```python
from build123d import *

# Parameters (mm, degrees)
SKETCH1_R               = 25
BOSS_EXTRUDE2_DEPTH     = 3.25
SKETCH2_R               = 4.5
BOSS_EXTRUDE3_DEPTH     = 10
SKETCH3_R               = 4.5
BOSS_EXTRUDE4_DEPTH     = 5
SKETCH4_R               = 3.1
CUT_EXTRUDE1_DEPTH      = 2.5
SKETCH6_R               = 1.875
CUT_EXTRUDE2_DEPTH      = 1
CUT_EXTRUDE2_DEPTH_BACK = 19.25


with BuildPart() as part:
    # Sketch1 → Boss-Extrude2 (new body, symmetric)
    with BuildSketch(Plane.XY):
        Circle(SKETCH1_R)
    extrude(amount=BOSS_EXTRUDE2_DEPTH, both=True)

    # Sketch2 → Boss-Extrude3 (add)
    with BuildSketch(Plane.XY):
        Circle(SKETCH2_R)
    extrude(amount=BOSS_EXTRUDE3_DEPTH)

    # Sketch3 → Boss-Extrude4 (add)
    with BuildSketch(Plane(origin=(0, 0, -3.25), x_dir=(-1, 0, 0), z_dir=(0, 0, -1))):
        Circle(SKETCH3_R)
    extrude(amount=BOSS_EXTRUDE4_DEPTH)

    # Sketch4 → Cut-Extrude1 (cut)
    with BuildSketch(Plane(origin=(0, 0, -8.25), x_dir=(-1, 0, 0), z_dir=(0, 0, -1))):
        Circle(SKETCH4_R)
    extrude(amount=-CUT_EXTRUDE1_DEPTH, mode=Mode.SUBTRACT)

    # Sketch6 → Cut-Extrude2 (cut, two sides)
    with BuildSketch(Plane.XY.offset(10)) as cut_extrude2_sk:
        Circle(SKETCH6_R)
    extrude(amount=CUT_EXTRUDE2_DEPTH, mode=Mode.SUBTRACT)
    extrude(cut_extrude2_sk.sketch, amount=-CUT_EXTRUDE2_DEPTH_BACK, mode=Mode.SUBTRACT)


solid = part.part
```
Design review of the part built by this model. Coordinates are the model's own, in mm. A direction names the side the tool comes from. Coordinates: 2 decimals unless noted, no trailing zeros. Write each loop counter-clockwise with the first axis right and the second up, starting at its lowest first coordinate (ties: lowest second). Pieces come first, ordered by that corner, then holes.
1) Add section A-A (x = 0). Write out the cut boundary in (y, z) (3 decimals), plus the area to 3 significant figures.
2) Machinability: for faces 1 (the flat face through (-1, -2, -5.75)), 2 (the cylindrical face through (23.846, 7.509, 0.046)), which of the approach directions +Z, -Z, +X, -X, +Y, -Y give a long, thin tool a straight path to every point of the face, cutting with its end or side? Answer none if there is none.
3) Insertion check: pin 1 (1 mm diameter, centred on y = -17.5, z = -3.5, fed in from -X); pin 2 (1.5 mm diameter, centred on x = -20, z = -5, fed in from +Y); pin 3 (5 mm diameter, centred on x = 0, y = 0, fed in from -Z); pin 4 (1.5 mm diameter, centred on y = -6, z = -2, fed in from +X). Each pin has a flat end and moves straight along its axis. Give the tip position at first contact, or say it passes through.
4) To check wall thickness, follow L1, parallel to Y at x = 0, z = -7.3; L2, parallel to Y at x = 0, z = 2.5 (3 decimals); L3, parallel to Z at x = 13, y = -4. State the ranges of each line that lie inside material, in increasing order.
5) Mouldability with a two-part tool opening along Y and no side actions: class faces 3 (the flat face through (0, -5, -3.25)), 4 (the cylindrical face through (-1.873, 0.082, 2.235)), 5 (the cylindrical face through (-0.59, 4.46, 6.58)) as +Y half, -Y half, draft (parallel to the pull), parting line (faces both ways), or undercut.
6) Add section C-C (z = -2.5). Write out the cut boundary in (x, y) (3 decimals), plus the area to 3 significant figures.
7) Add section D-D (x = -20). Write out the cut boundary in (y, z), plus the area to 3 significant figures.
Check result:
1. outline: (-25, -3.25) - (-4.5, -3.25) - (-4.5, -8.25) - (-3.1, -8.25) - (-3.1, -5.75) - (-1.875, -5.75) - (-1.875, 10) - (-4.5, 10) - (-4.5, 3.25) - (-25, 3.25) - close; (1.875, -5.75) - (3.1, -5.75) - (3.1, -8.25) - (4.5, -8.25) - (4.5, -3.25) - (25, -3.25) - (25, 3.25) - (4.5, 3.25) - (4.5, 10) - (1.875, 10) - close
1. area: 356 mm2
2. face 1: -Z
2. face 2: +Z, -Z
3. pin 1: stops at x = -18.27
3. pin 2: passes through
3. pin 3: stops at z = -5.75
3. pin 4: stops at x = 24.44
4. L1: y = -4.5 to -3.1, 3.1 to 4.5
4. L2: y = -25 to -1.875, 1.875 to 25
4. L3: z = -3.25 to 3.25
5. face 3: draft
5. face 4: undercut
5. face 5: parting line
6. outline: circle Ø50 at (0, 0); hole circle Ø3.75 at (0, 0)
6. area: 1,950 mm2
7. outline: (-15, -3.25) - (15, -3.25) - (15, 3.25) - (-15, 3.25) - close
7. area: 195 mm2
